Here's how the part is built. I have some questions about the finished solid (model axes, mm). A direction names the side the tool comes from. Round coordinates to 2 decimals unless told otherwise and drop trailing zeros. Write each loop counter-clockwise with the first axis right and the second up, starting at its lowest first coordinate (ties: lowest second). Pieces come first, ordered by that corner, then holes. Notation, with made-up numbers: (20, 36) -> (73, 36) arc R21 cw to (73, 62) -> close; hole circle Ø9 at (83.25, 42.5). An arc over 180 degrees is marked (long way). Put each result on its own line as item: value. Start each with the question number.
1) I want a section at C-C, the plane z = 0.3. List the corners of the cut face in (x, y) for me, then the cut area to 3 significant figures.
2) Which directions (+Z, -Z, +X, -X, +Y, -Y) give clear straight access to the entire face, cutting with the end or side of a thin tool? Please do faces 1 (the flat face through (6.9, 8.574, 0.5)), 2 (the flat face through (7, 8, 1)).
3) I want a section at B-B, the plane y = 10.05. List the corners of the cut face in (x, z) for me, then the cut area to 3 significant figures.
4) I want a section at A-A, the plane x = 6. List the corners of the cut face in (y, z) for me, then the cut area to 3 significant figures.
5) If I drill on line 1 along X through (y, z) = (10.65, 0.7); line 2 along Y through (x, z) = (3.25, 0.9), over which ranges is the centre line in solid material (lowest first)? Write a range as [from, to].
6) We'd pull the mould along Y, two halves only. Please class faces 3 (the flat face through (6.9, 7.602, 0.5)), 4 (the flat face through (1.272, 9.7, 0.5)), 5 (the flat face through (6.7, 10.896, 0.5)), 6 (the flat face through (7, 8, 0)): released by +Y, released by -Y, zero draft, split by the parting line, or undercut.
Autodesk Inventor part; units mm, degrees
ref_plane "YZ Plane" through (0, 0, 0) normal (1, 0, 0) x (0, 1, 0)
ref_plane "XZ Plane" through (0, 0, 0) normal (0, 1, 0) x (-1, 0, 0)
ref_plane "XY Plane" through (0, 0, 0) normal (0, 0, 1) x (1, 0, 0)
sketch "Sketch1" plane through (0, 0, 0) normal (0, 0, 1) x (1, 0, 0)
  line L0 (0, 11.9936) -> (13.6628, 11.9936)
  line L1 (13.6628, 11.9936) -> (13.6628, 7.6017)
  line L2 (13.6628, 7.6017) -> (0, 7.6017)
  line L3 (0, 7.6017) -> (0, 11.9936)
  line L4 (1.2716, 10.8956) -> (12.3453, 10.8956)
  line L5 (12.3453, 10.8956) -> (12.3453, 8.5742)
  line L6 (12.3453, 8.5742) -> (1.2716, 8.5742)
  line L7 (1.2716, 8.5742) -> (1.2716, 10.8956)
  point P0 (0, 0)
extrude "Extrusion1" add sketch "Sketch1" along normal blind 1
properties part number "lcd1"
Findings:
1. outline: (0, 7.6) -> (13.66, 7.6) -> (13.66, 11.99) -> (0, 11.99) -> close; hole (1.27, 8.57) -> (12.35, 8.57) -> (12.35, 10.9) -> (1.27, 10.9) -> close
1. area: 34.3 mm2
2. face 1: +Z, -Z
2. face 2: +Z, +X, -X, +Y, -Y
3. outline: (0, 0) -> (1.27, 0) -> (1.27, 1) -> (0, 1) -> close; (12.35, 0) -> (13.66, 0) -> (13.66, 1) -> (12.35, 1) -> close
3. area: 2.59 mm2
4. outline: (7.6, 0) -> (8.57, 0) -> (8.57, 1) -> (7.6, 1) -> close; (10.9, 0) -> (11.99, 0) -> (11.99, 1) -> (10.9, 1) -> close
4. area: 2.07 mm2
5. line 1: x = [0, 1.27], [12.35, 13.66]
5. line 2: y = [7.6, 8.57], [10.9, 11.99]
6. face 3: released by -Y
6. face 4: undercut
6. face 5: undercut
6. face 6: zero draft
